Check sheet for the drawn part. Datum: minimum x, y, z corner. Units: mm. A direction names the side the tool comes from. Coordinates: 2 decimals unless noted, no trailing zeros. Loops run counter-clockwise (first coordinate to the right, second up) from the corner with the lowest first, then second, coordinate; pieces in that order, holes last.
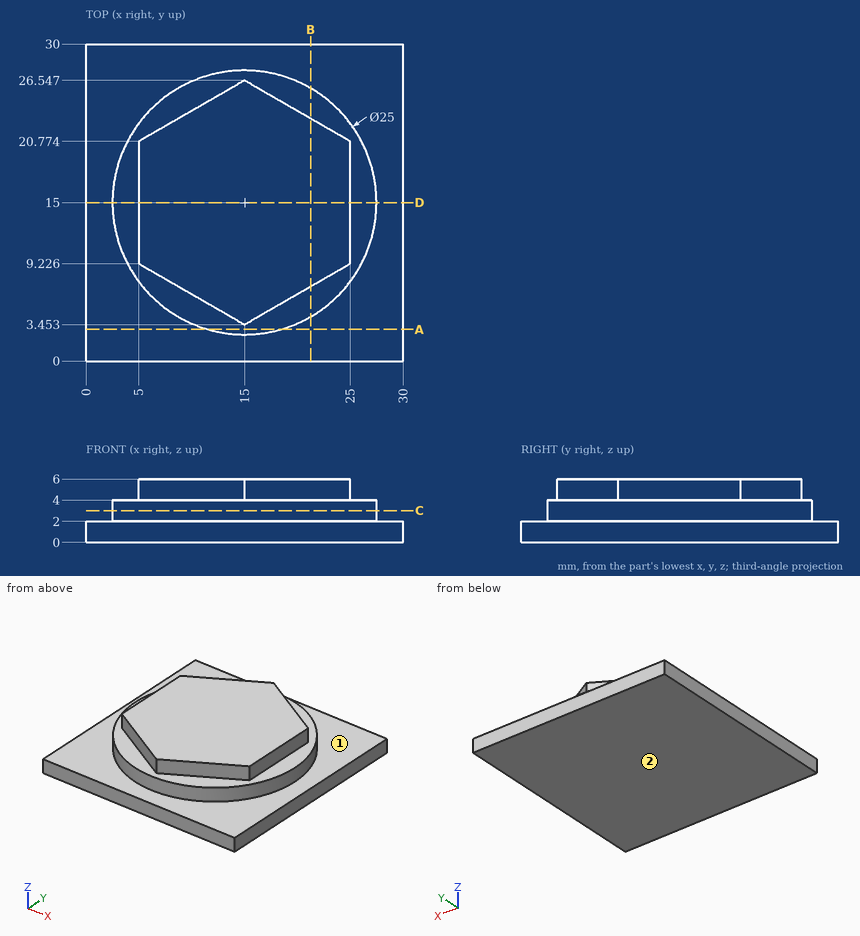
1) Set-up check for the marked faces 1 and 2: record each of +Z, -Z, +X, -X, +Y, -Y from which the full face is reachable in a straight line by a thin tool's end or side.
Answer sheet:
face 1: +Z
face 2: -Z, +X, -X, +Y, -Y
2) Section check A-A on y = 3. Enter the section's corners in (x, z).
Answer sheet:
outline: (0, 0) - (30, 0) - (30, 2) - (18.5, 2) - (18.5, 4) - (11.5, 4) - (11.5, 2) - (0, 2) - close
3) Section check D-D on y = 15. Enter the section's corners in (x, z), plus the area to 3 significant figures.
Answer sheet:
outline: (0, 0) - (30, 0) - (30, 2) - (27.5, 2) - (27.5, 4) - (25, 4) - (25, 6) - (5, 6) - (5, 4) - (2.5, 4) - (2.5, 2) - (0, 2) - close
area: 150 mm2
4) Section check C-C on z = 3. Enter the section's corners in (x, y).
Answer sheet:
outline: circle Ø25 at (15, 15)
5) Scan lines: line 1 (Z direction, x = 10.75, y = 28); line 2 (Z direction, x = 24.25, y = 23); line 3 (X direction, y = 14, z = 4.9). Record each from-to range of solid material in increasing order.
Answer sheet:
line 1: z = 0 to 2
line 2: z = 0 to 4
line 3: x = 5 to 25
6) Section check B-B on x = 21.25. Enter the section's corners in (y, z) (1 decimal), plus the area to 3 significant figures.
Answer sheet:
outline: (0, 0) - (30, 0) - (30, 2) - (25.8, 2) - (25.8, 4) - (22.9, 4) - (22.9, 6) - (7.1, 6) - (7.1, 4) - (4.2, 4) - (4.2, 2) - (0, 2) - close
area: 135 mm2
7) Depth check by flat-ended pin: pin 1 (2 mm diameter, centred on y = 11.5, z = 3.5, fed in from -X); pin 2 (2 mm diameter, centred on y = 13.5, z = 4.5, fed in from -X); pin 3 (2 mm diameter, centred on y = 13.5, z = 5.5, fed in from +X). Enter the tip coordinate at first touch or a pass-through.
Answer sheet:
pin 1: stops at x = 2.75
pin 2: stops at x = 2.52
pin 3: stops at x = 25
